from build123d import *

# Parameters (mm, degrees)
F0_W     = 2.5
F0_H     = 3
F2_R     = 2.5
F3_DEPTH = 4
F7_D     = 3.3
F7_DEPTH = 3
F7_TIP   = 0.9914200214
F9_D     = 0.4


with BuildPart() as f1:
    # F0 (on Front) → F1 (revolve)
    with BuildSketch(Plane.XZ):
        with Locations((1.25, 1.5)):
            Rectangle(F0_W, F0_H)
    revolve(axis=Axis((0, 0, 1.5), (0, 0, 1)))

    # F2 (on face) → F3 (join)
    with BuildSketch(Plane(origin=(0, 0, 0), x_dir=(1, 0, 0), z_dir=(0, 0, -1))):
        Polygon((1.7320508076, 3), (-1.7320508076, 3), (-3.4641016151, 0), (-1.7320508076, -3), (1.7320508076, -3), (3.4641016151, 0), align=None)
        Circle(F2_R, mode=Mode.SUBTRACT)
        Circle(F2_R)
    extrude(amount=F3_DEPTH)

    # F4 (on Front) → F5 (revolve)
    with BuildSketch(Plane.XZ):
        Polygon((2, -4), (0, -4), (0, -6), align=None)
    revolve(axis=Axis((0, 0, -5), (0, 0, 1)))

    # F7
    with Locations(Plane.XY.offset(3)):
        with Locations((0, 0)):
            Hole(F7_D / 2, depth=F7_DEPTH)
            with Locations((0, 0, -(F7_DEPTH + F7_TIP / 2))):  # 118° drill point
                Cone(0, F7_D / 2, F7_TIP, mode=Mode.SUBTRACT)

    # F9 (through all)
    with Locations(Plane.XY.offset(3)):
        with Locations((0, 0)):
            Hole(F9_D / 2)


solid = f1.part
Source: CAD feature listing. Evaluate the final solid. Frame: model axes, mm. A direction names the side the tool comes from. Give positions to 0.01 mm unless a question says otherwise; leave off trailing zeros. Write each loop counter-clockwise with the first axis right and the second up, starting at its lowest first coordinate (ties: lowest second). Pieces come first, ordered by that corner, then holes. Notation, with made-up numbers: M 60,45.25 L 92,45.25 A25 ccw 92,76.25 Z; hole C 10.5,75.5 d1. An arc over 180 degrees is marked long. Return JSON: item names as keys, results as strings. Group by question number.
1) Cut plane B-B, the plane x = 0. Output: boundary loops of the cut face in (y, z), then the cut area to 3 significant figures.
2) Draft query along Y for faces 4 (the face through (2.6, 1.5, -2)), 5 (the face through (0.49, 0.15, -5.49)), 6 (the face through (1.216, 1.115, 1.479)), 7 (the face through (2.6, -1.5, -2)). Return one class per face: released by +Y, released by -Y, zero draft, split by the parting line, or undercut.
3) Cut plane D-D, the plane x = 3. Output: boundary loops of the cut face in (y, z).
4) Cut plane A-A, the plane z = -2. Output: boundary loops of the cut face in (x, y), then the cut area to 3 significant figures.
5) Cut plane C-C, the plane z = -5. Output: boundary loops of the cut face in (x, y).
6) Ray query, L1, parallel to Y at x = 0, z = -3.4; L2, parallel to Y at x = 0, z = 1.4; L3, parallel to Z at x = 1.75, y = -1.25. Return the intervals inside material, ascending.
7) First-contact query: pin 1 Ø3 at (x, y) = (0, 0) entering from +Z. Flat tip, straight axial feed; report the tip coordinate or a pass-through.
8) Set-up query: faces 1 (the face through (0, 3, -2)), 2 (the face through (-0.54, -2.44, 1.52)), 3 (the face through (1, -2, -4)). Return all of +Z, -Z, +X, -X, +Y, -Y with unobstructed straight access to the full face (end or side cutting, diameter ignored); none if empty.
Data:
{
 "1": {"outline": "M -3,-4 L -2,-4 L -0.2,-5.8 L -0.2,-0.87 L -1.65,0 L -1.65,3 L -2.5,3 L -2.5,0 L -3,0 Z; M 0.2,-5.8 L 2,-4 L 3,-4 L 3,0 L 2.5,0 L 2.5,3 L 1.65,3 L 1.65,0 L 0.2,-0.87 Z", "area": "29.5 mm²"},
 "2": {"face 4": "released by +Y", "face 5": "split by the parting line", "face 6": "undercut", "face 7": "released by -Y"},
 "3": {"outline": "M -0.8,-4 L 0.8,-4 L 0.8,0 L -0.8,0 Z"},
 "4": {"outline": "M -3.46,0 L -1.73,-3 L 1.73,-3 L 3.46,0 L 1.73,3 L -1.73,3 Z; hole C 0,0 d0.4", "area": "31.1 mm²"},
 "5": {"outline": "C 0,0 d2; hole C 0,0 d0.4"},
 "6": {"L1": "y = -3 to -0.2, 0.2 to 3", "L2": "y = -2.5 to -1.65, 1.65 to 2.5", "L3": "z = -4 to 3"},
 "7": {"pin 1": "stops at z = -0.09"},
 "8": {"face 1": "+Z, -Z, +X, -X, +Y", "face 2": "+Z", "face 3": "-Z"}
}
